Check sheet for the drawn part. Datum: minimum x, y, z corner. Units: mm. Give positions to 0.01 mm unless a question says otherwise; leave off trailing zeros. Loops run counter-clockwise (first coordinate to the right, second up) from the corner with the lowest first, then second, coordinate; pieces in that order, holes last. Notation, with made-up numbers: (21, 21) - (61, 21) arc R9 ccw to (61, 38) - close; hole circle Ø10 at (-32, 26). An arc over 180 degrees is marked (long way). Use a Markdown table: item, result. Add a question column.
1. Material ranges on L1, parallel to Z at x = 14.5, y = 12.5; L2, parallel to Z at x = 8, y = 10.75; L3, parallel to X at y = 14, z = 421, recorded low to high.
2. Cross-section at C-C on x = 18.25. Enter the section's corners in (y, z), and give its area (3 significant figures).
3. Depth check by flat-ended pin: P1, Ø12, axis at x = 11, z = 526, coming from the -Y side; P2, Ø1, axis at x = 14, z = 83, coming from the +Y side; P3, Ø5, axis at x = 5.5, z = 141.5, coming from the -Y side; P4, Ø3, axis at x = 5.5, z = 407, coming from the -Y side. Enter the tip coordinate at first touch or a pass-through.
4. Cross-section at D-D on z = 359.5. Enter the section's corners in (x, y).
5. Cross-section at B-B on z = 450. Enter the section's corners in (x, y), and give its area (3 significant figures).
6. Cross-section at A-A on y = 12.7. Enter the section's corners in (x, z), and give its area (3 significant figures).
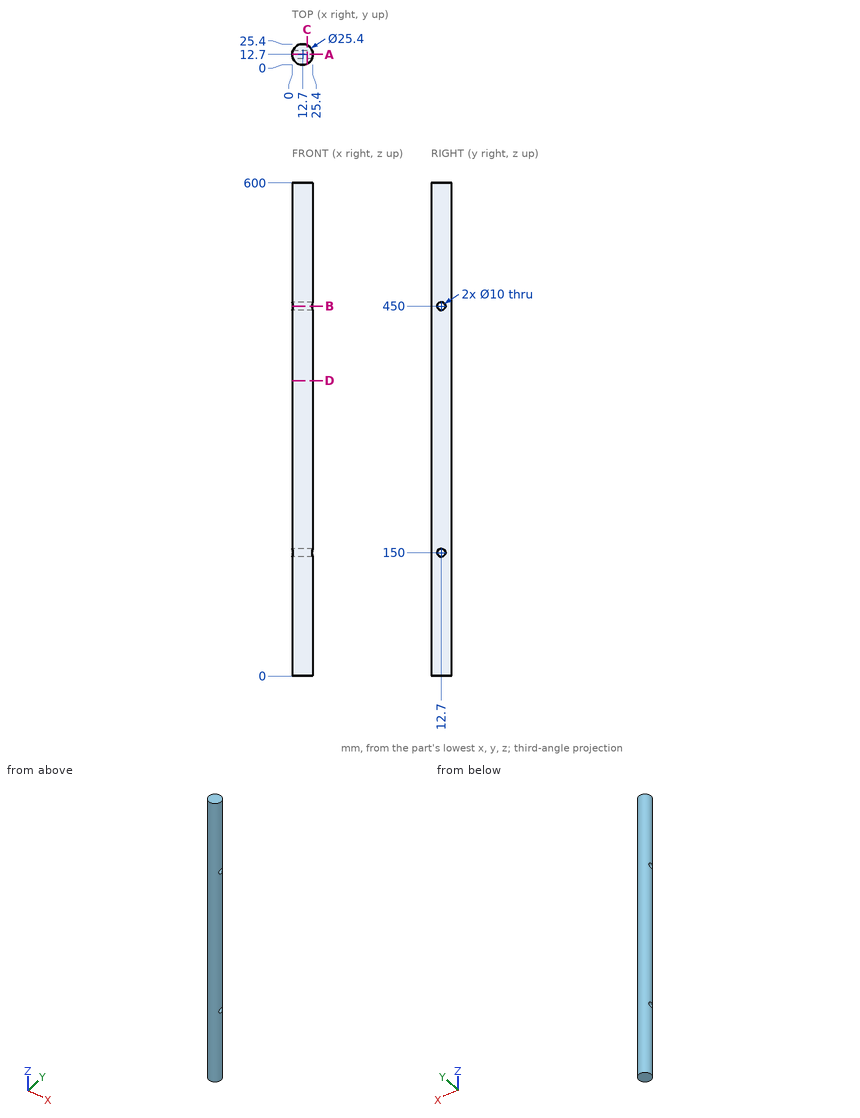
Values found:
| question | item | result |
|---|---|---|
| 1 | L1 | z = 0 to 145, 155 to 445, 455 to 600 |
| 1 | L2 | z = 0 to 145.4, 154.6 to 445.4, 454.6 to 600 |
| 1 | L3 | x = 0.07 to 25.33 |
| 2 | outline | (1.28, 0) - (24.12, 0) - (24.12, 600) - (1.28, 600) - close; hole circle Ø10 at (12.7, 150); hole circle Ø10 at (12.7, 450) |
| 2 | area | 13,600 mm2 |
| 3 | P1 | stops at y = 0 |
| 3 | P2 | stops at y = 25.37 |
| 3 | P3 | stops at y = 0.9 |
| 3 | P4 | stops at y = 1.35 |
| 4 | outline | circle Ø25.4 at (12.7, 12.7) |
| 5 | outline | (1.03, 7.7) arc R12.7 ccw to (24.37, 7.7) - close; (1.03, 17.7) - (24.37, 17.7) arc R12.7 ccw to start |
| 5 | area | 259 mm2 |
| 6 | outline | (0, 0) - (25.4, 0) - (25.4, 145) - (0, 145) - close; (0, 155) - (25.4, 155) - (25.4, 445) - (0, 445) - close; (0, 455) - (25.4, 455) - (25.4, 600) - (0, 600) - close |
| 6 | area | 14,700 mm2 |
